For this review, use the dimensioned drawing (mm, ordinates from the lowest corner) and the shaded views. Coordinates: 2 decimals unless noted, no trailing zeros. Write each loop counter-clockwise with the first axis right and the second up, starting at its lowest first coordinate (ties: lowest second). Pieces come first, ordered by that corner, then holes. Notation, with made-up numbers: (-34.5, 40.5) -> (7.5, 40.5) arc R22 cw to (7.5, 58.5) -> close; hole circle Ø6 at (44.25, 35). An arc over 180 degrees is marked (long way). Return JSON: item names as keys, results as strings. Group by question number.
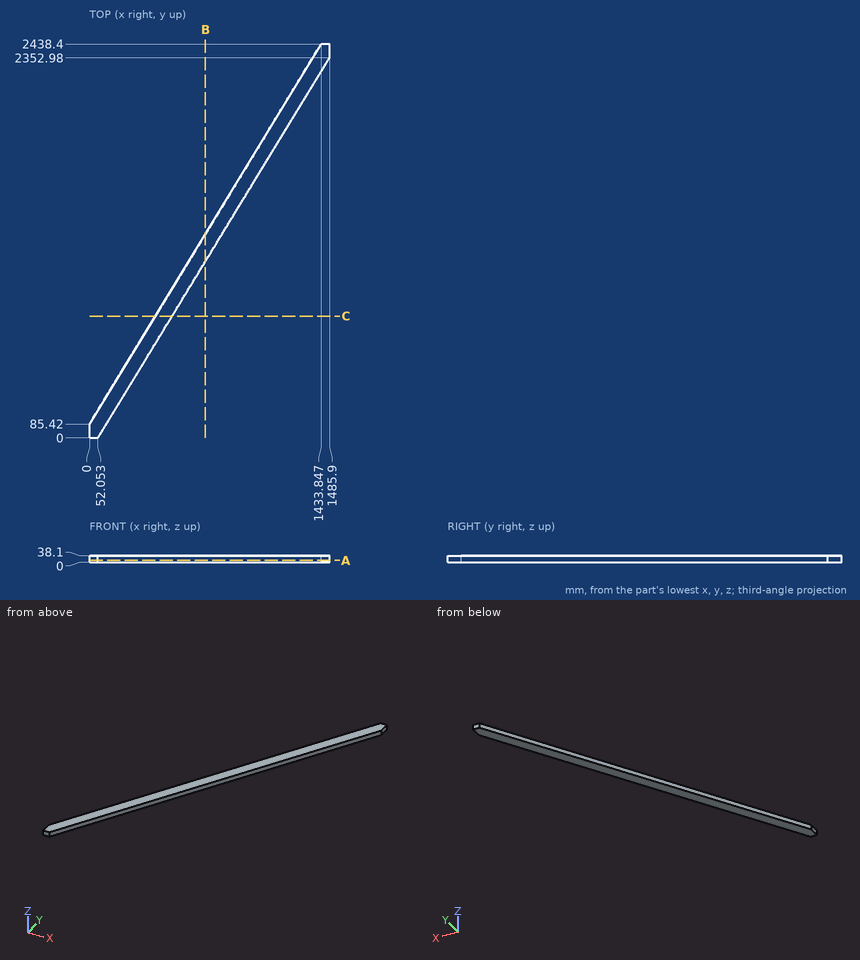
Q1. For P1, Ø2, axis at x = 778, z = 11.5, coming from the -Y side; P2, Ø8, axis at x = 876, z = 7, coming from the -Y side (1 decimal); P3, Ø3, axis at y = 1305, z = 29, coming from the -X side, all flat-tipped, find the tip position at first contact; note any pin that passes through.
Q2. We need section B-B on x = 717.5. Write out the cut boundary in (y, z), plus the area to 3 significant figures.
Q3. Wall thickness on L1, parallel to Y at x = 1265, z = 28.5; L2, parallel to X at y = 1865, z = 16; L3, parallel to X at y = 497, z = 23.5: over which ranges is each line inside the solid? List them lowest first.
Q4. We need section C-C on y = 753.5. Write out the cut boundary in (x, z).
Q5. We need section A-A on z = 11. Write out the cut boundary in (x, y), plus the area to 3 significant figures.
Findings below:
{
 "1": {"P1": "stops at y = 1189.66", "P2": "stops at y = 1345.6", "P3": "stops at x = 742.27"},
 "2": {"outline": "(1092.02, 0) -> (1262.86, 0) -> (1262.86, 38.1) -> (1092.02, 38.1) -> close", "area": "6,510 mm^2"},
 "3": {"L1": "y = 1990.48 to 2161.32", "L2": "x = 1084.43 to 1188.54", "L3": "x = 250.81 to 354.91"},
 "4": {"outline": "(407.11, 0) -> (511.22, 0) -> (511.22, 38.1) -> (407.11, 38.1) -> close"},
 "5": {"outline": "(0, 0) -> (52.05, 0) -> (1485.9, 2352.98) -> (1485.9, 2438.4) -> (1433.85, 2438.4) -> (0, 85.42) -> close", "area": "249,000 mm^2"}
}
